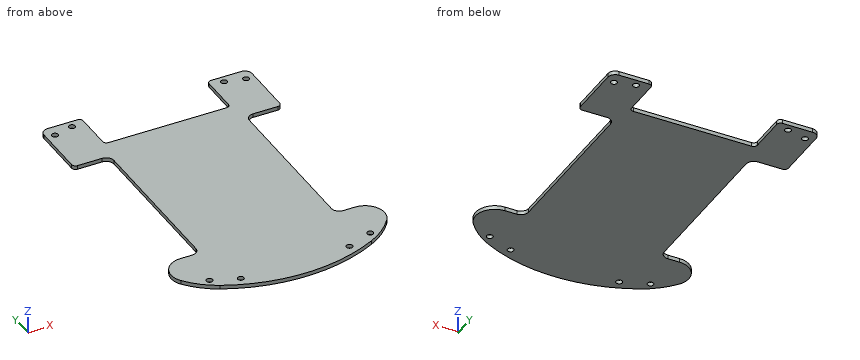
from build123d import *

# Parameters (mm, degrees)
SKETCH1_R                = 1.6
BOSS_EXTRUDE1_DEPTH      = 2
M3_CLEARANCE_HOLE1_D     = 3.2
M3_CLEARANCE_HOLE1_DEPTH = 2
M3_CLEARANCE_HOLE1_TIP   = 0.96137699


with BuildPart() as part:
    # Sketch1 → Boss-Extrude1 (new body)
    with BuildSketch(Plane(origin=(0, 0, 0), x_dir=(-1, 0, 0), z_dir=(0, 0, -1))):
        with BuildLine():
            Line((49.999999993, 71.749999992), (34.499999968, 71.749999992))
            ThreePointArc((34.499999968, 71.749999992), (33.085786407, 71.164213555), (32.49999997, 69.749999994))
            Line((32.49999997, 69.749999994), (32.49999997, 50.749999994))
            ThreePointArc((32.49999997, 50.749999994), (31.914213535, 49.335786439), (30.49999998, 48.750000004))
            Line((30.49999998, 48.750000004), (-30.50000002, 48.750000004))
            ThreePointArc((-30.50000002, 48.750000004), (-31.914213575, 49.335786439), (-32.50000001, 50.749999994))
            Line((-32.50000001, 50.749999994), (-32.50000001, 69.749999994))
            ThreePointArc((-32.50000001, 69.749999994), (-33.085786447, 71.164213555), (-34.500000007, 71.749999992))
            Line((-34.500000007, 71.749999992), (-50.000000007, 71.749999992))
            ThreePointArc((-50.000000007, 71.749999992), (-52.651650433, 70.651650422), (-53.750000002, 67.999999996))
            Line((-53.750000002, 67.999999996), (-53.750000002, 40.749999996))
            ThreePointArc((-53.750000002, 40.749999996), (-53.164213571, 39.335786449), (-51.750000024, 38.750000018))
            Line((-51.750000024, 38.750000018), (-39.000000024, 38.750000018))
            ThreePointArc((-39.000000024, 38.750000018), (-36.171572886, 37.578427137), (-35.000000005, 34.75))
            Line((-35.000000005, 34.75), (-35.000000005, -46))
            ThreePointArc((-35.000000005, -46), (-36.171572879, -48.828427121), (-38.999999999, -49.999999994))
            Line((-38.999999999, -49.999999994), (-45.09502308, -49.999999994))
            ThreePointArc((-45.09502308, -49.999999994), (-54.039294999, -55.527864046), (-53.095023084, -66.000000011))
            ThreePointArc((-53.095023084, -66.000000011), (-46.752677079, -72.686883058), (-39.048234252, -77.744680848))
            ThreePointArc((-39.048234252, -77.744680848), (1.5e-08, -86.999999997), (39.048234283, -77.744680848))
            ThreePointArc((39.048234283, -77.744680848), (46.752677109, -72.686883058), (53.095023115, -66.000000011))
            ThreePointArc((53.095023115, -66.000000011), (54.039295029, -55.527864046), (45.095023111, -49.999999994))
            Line((45.095023111, -49.999999994), (39.000000001, -49.999999994))
            ThreePointArc((39.000000001, -49.999999994), (36.17157288, -48.828427121), (35.000000007, -46))
            Line((35.000000007, -46), (35.000000007, 34.75))
            ThreePointArc((35.000000007, 34.75), (36.171572888, 37.578427137), (39.000000025, 38.750000018))
            Line((39.000000025, 38.750000018), (51.750000009, 38.750000018))
            ThreePointArc((51.750000009, 38.750000018), (53.164213556, 39.335786449), (53.749999988, 40.749999996))
            Line((53.749999988, 40.749999996), (53.749999988, 67.999999996))
            ThreePointArc((53.749999988, 67.999999996), (52.651650419, 70.651650422), (49.999999993, 71.749999992))
        make_face()
        with Locations((49.348831914, 65.488111827)):
            Circle(SKETCH1_R, mode=Mode.SUBTRACT)
        with Locations((-49.348831883, 65.488111827)):
            Circle(SKETCH1_R, mode=Mode.SUBTRACT)
        with Locations((28.045651768, -77.054794901)):
            Circle(SKETCH1_R, mode=Mode.SUBTRACT)
        with Locations((-28.045651737, -77.054794901)):
            Circle(SKETCH1_R, mode=Mode.SUBTRACT)
    extrude(amount=-BOSS_EXTRUDE1_DEPTH)

    # M3 Clearance Hole1
    with Locations(Plane(origin=(-39.259818305, 68, 2), x_dir=(1, 0, 0), z_dir=(0, 0, 1))):
        with Locations((0, 0), (78.51963661, 0), (80.759818305, -139.880108514), (-2.240181695, -139.880108514)):
            Hole(M3_CLEARANCE_HOLE1_D / 2, depth=M3_CLEARANCE_HOLE1_DEPTH)
            with Locations((0, 0, -(M3_CLEARANCE_HOLE1_DEPTH + M3_CLEARANCE_HOLE1_TIP / 2))):  # 118° drill point
                Cone(0, M3_CLEARANCE_HOLE1_D / 2, M3_CLEARANCE_HOLE1_TIP, mode=Mode.SUBTRACT)


solid = part.part
Input: part model. Units: mm. Frame: model coordinates. Give positions to 0.01 mm unless a question says otherwise; leave off trailing zeros. Order: outer loops, then holes, each group sorted by start corner. A loop starts at its lowest first (then second) coordinate and runs counter-clockwise, first axis right, second up.
Q1. Section B-B on y = -42.5. Output: boundary loops of the cut face in (x, z).
Checked values:
outline: (-35, 0) - (35, 0) - (35, 2) - (-35, 2) - close
Q2. Ray query, probe 1 along X at (y, z) = (68, 0.8); probe 2 along Y at (x, z) = (38.5, 0.35); probe 3 along Y at (x, z) = (-48.5, 0.55). Return the intervals inside material, ascending.
Checked values:
probe 1: x = -53.75 to -40.86, -37.66 to -32.5, 32.5 to 37.66, 40.86 to 53.75
probe 2: y = -78.02 to -49.97, 38.72 to 66.59, 69.41 to 71.75
probe 3: y = -71.14 to -50.6, 38.75 to 64.13, 66.84 to 71.75
Q3. Section A-A on y = 54.5. Output: boundary loops of the cut face in (x, z).
Checked values:
outline: (-53.75, 0) - (-32.5, 0) - (-32.5, 2) - (-53.75, 2) - close; (32.5, 0) - (53.75, 0) - (53.75, 2) - (32.5, 2) - close
Q4. Section D-D on z = 0.85. State how many separate pieces and enclosed holes the cut face has, and give its area (3 significant figures).
Checked values:
separate pieces: 1
enclosed holes: 8
area: 11,500 mm2
Q5. Contact query for flat-ended pins moving along their axis: pin 1 Ø0.6 at (y, z) = (50.5, 1) entering from +X; pin 2 Ø1 at (y, z) = (57.5, 1) entering from -X; pin 3 Ø2.5 at (x, y) = (41.5, -71.88) entering from -Z; pin 4 Ø1 at (y, z) = (-25.5, 1.5) entering from -X. Output: stop coordinate, or through.
Checked values:
pin 1: stops at x = 53.75
pin 2: stops at x = -53.75
pin 3: passes through
pin 4: stops at x = -35
Q6. Section C-C on x = 23.5. Output: boundary loops of the cut face in (y, z).
Checked values:
outline: (-83.77, 0) - (48.75, 0) - (48.75, 2) - (-83.77, 2) - close
